Check sheet for the modelled part. Datum: model origin and axes. Units: mm. Face numbers are marked on the shaded views. Give positions to 0.01 mm unless a question says otherwise; leave off trailing zeros. Write each loop counter-clockwise with the first axis right and the second up, starting at its lowest first coordinate (ties: lowest second). Pieces come first, ordered by that corner, then holes. Notation, with made-up numbers: M 45.5,-30.75 L 57.5,-30.75 A23 ccw 57.5,7.25 Z; hole C -1.5,32.25 d9. An arc over 180 degrees is marked long. Use CSV: the item, a comma, the result in double quotes. Start each with the question number.
1. Depth check by flat-ended pin: P1, Ø2, axis at x = -35, y = -8.5, coming from the -Z side; P2, Ø1, axis at y = -6.5, z = 16.5, coming from the +X side; P3, Ø8, axis at y = -18.5, z = 5, coming from the -X side. Enter the tip coordinate at first touch or a pass-through.
2. Scan lines: line 1 (X direction, y = -22.75, z = 23.5); line 2 (X direction, y = -14.25, z = 21); line 3 (X direction, y = -17.5, z = 11.5). Record each from-to range of solid material in increasing order.
3. Cross-section at B-B, the plane y = -10.5. Enter the section's corners in (x, z) (1 decimal).
4. Cross-section at D-D, the plane z = 6. Enter the section's corners in (x, y).
5. Cross-section at C-C, the plane x = -35. Enter the section's corners in (y, z), and give its area (3 significant figures).
6. Mould release check, pull along X, two halves, no side actions. Record for the marked faces 1, 2 and 3: +X half, -X half, draft (parallel to the pull), parting line (faces both ways), or undercut.
7. Cross-section at A-A, the plane z = 22.5. Enter the section's corners in (x, y), and give its area (3 significant figures).
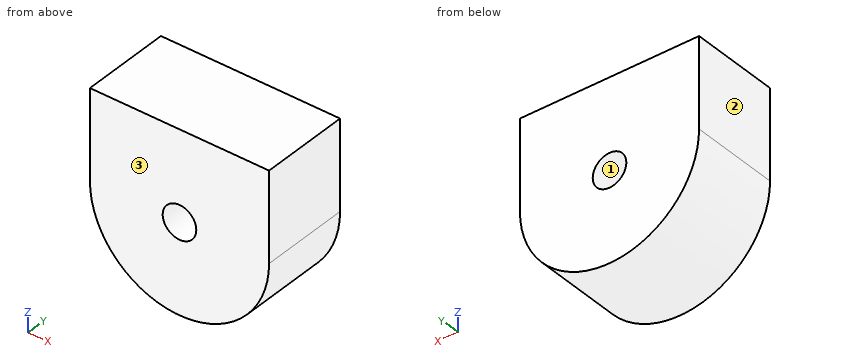
from build123d import *

# Parameters (mm, degrees)
F0_R     = 4.7625
F1_DEPTH = 25.4


with BuildPart() as f1:
    # F0 (on Front) → F1 (new body)
    with BuildSketch(Plane.XZ):
        with BuildLine():
            ThreePointArc((-72.612513, 23.634593), (-47.212513, -1.765407), (-21.812513, 23.634593))
            Line((-21.812513, 23.634593), (-21.812513, 49.034593))
            Line((-21.812513, 49.034593), (-72.612513, 49.034593))
            Line((-72.612513, 49.034593), (-72.612513, 23.634593))
        make_face()
        with Locations((-47.212513, 23.634593)):
            Circle(F0_R, mode=Mode.SUBTRACT)
    extrude(amount=F1_DEPTH)


solid = f1.part
Worked answers:
1,P1,"stops at z = 0.84"
1,P2,"stops at x = -22.69"
1,P3,"stops at x = -67.97"
2,line 1,"x = -72.61 to -51.97, -42.45 to -21.81"
2,line 2,"x = -72.48 to -51.18, -43.25 to -21.95"
2,line 3,"x = -69.53 to -24.9"
3,outline,"M -72.6,23.6 A25.4 ccw -21.8,23.6 L -21.8,49 L -72.6,49 Z; hole C -47.2,23.6 d9.5"
4,outline,"M -65.49,-25.4 L -28.93,-25.4 L -28.93,0 L -65.49,0 Z"
5,outline,"M -25.4,1.36 L 0,1.36 L 0,49.03 L -25.4,49.03 Z"
5,area,"1,210 mm^2"
6,face 1,"undercut"
6,face 2,"-X half"
6,face 3,"draft"
7,outline,"M -72.59,-25.4 L -51.84,-25.4 L -51.84,0 L -72.59,0 Z; M -42.59,-25.4 L -21.84,-25.4 L -21.84,0 L -42.59,0 Z"
7,area,"1,050 mm^2"
